Source: CAD feature listing. Evaluate the final solid. Frame: model axes, mm. A direction names the side the tool comes from. Give positions to 0.01 mm unless a question says otherwise; leave off trailing zeros. Loops run counter-clockwise (first coordinate to the right, second up) from the corner with the lowest first, then second, coordinate; pieces in that order, holes last. Notation, with made-up numbers: M -12.5,18 L 9.5,18 A14 cw 9.5,38 Z; hole C 86,29.25 d11. An arc over 180 degrees is marked long. Write item = value, one per line.
from build123d import *

# Parameters (mm, degrees)
BOSS_EXTRUDE1_DEPTH     = 13
SKETCH6_W               = 6
SKETCH6_H               = 5
BOSS_EXTRUDE4_DEPTH     = 5.6
SKETCH16_W              = 6
SKETCH16_H              = 8
BOSS_EXTRUDE5_DEPTH     = 0.1
CUT_EXTRUDE6_DEPTH      = 4
CUT_EXTRUDE6_DEPTH_BACK = 3.6
SKETCH15_R              = 1.2
CUT_EXTRUDE7_DEPTH      = 8.7202
CUT_EXTRUDE8_START      = -0.2202
SKETCH19_W              = 6
SKETCH19_H              = 8
SKETCH19_R              = 1.2
CUT_EXTRUDE8_DEPTH      = 0.2202
SKETCH12_R              = 1.2
CUT_EXTRUDE5_DEPTH      = 6
CHAMFER1_SIZE           = 0.2
SKETCH21_R              = 1.2
BOSS_EXTRUDE6_DEPTH     = 2.5
SKETCH24_W              = 6
SKETCH24_H              = 5.5
CUT_EXTRUDE10_DEPTH     = 8.5
SKETCH25_W              = 6
SKETCH25_H              = 7
BOSS_EXTRUDE8_DEPTH     = 12.9
SKETCH26_W              = 6
SKETCH26_H              = 7.39
BOSS_EXTRUDE9_DEPTH     = 3
SKETCH30_R              = 1.2
CUT_EXTRUDE13_DEPTH     = 8
SKETCH31_W              = 7
SKETCH31_H              = 9
BOSS_EXTRUDE11_DEPTH    = 1
SKETCH32_W              = 7
SKETCH32_H              = 9
BOSS_EXTRUDE12_DEPTH    = 1
BOSS_EXTRUDE13_DEPTH    = 1
BOSS_EXTRUDE14_DEPTH    = 1
SKETCH35_W              = 10
SKETCH35_H              = 4.2
CUT_EXTRUDE14_DEPTH     = 10
BOSS_EXTRUDE15_DEPTH    = 6
SKETCH38_R              = 1.2
CUT_EXTRUDE15_DEPTH     = 4
SKETCH39_R              = 1.2
CUT_EXTRUDE16_DEPTH     = 10
SKETCH40_W              = 14
SKETCH40_H              = 1.5
CUT_EXTRUDE17_DEPTH     = 10
SKETCH41_W              = 6.5
SKETCH41_H              = 3.19
CUT_EXTRUDE18_DEPTH     = 1.5


with BuildPart() as part:
    # Sketch1 → Boss-Extrude1 (new body)
    with BuildSketch(Plane.XY):
        Polygon((3, 3.05), (3, -2.253801214), (2.388188946, -2.95), (-2.388188946, -2.95), (-3, -2.253801214), (-3, 3.05), align=None)
    extrude(amount=BOSS_EXTRUDE1_DEPTH)

    # Sketch6 → Boss-Extrude4 (add)
    with BuildSketch(Plane(origin=(0, 3.05, 0), x_dir=(1, 0, 0), z_dir=(0, 1, 0))):
        with Locations((0, -2.5)):
            Rectangle(SKETCH6_W, SKETCH6_H)
    extrude(amount=BOSS_EXTRUDE4_DEPTH)

    # Sketch16 → Boss-Extrude5 (add)
    with BuildSketch(Plane(origin=(0, 3.05, 0), x_dir=(1, 0, 0), z_dir=(0, 1, 0))):
        with Locations((0, -9)):
            Rectangle(SKETCH16_W, SKETCH16_H)
    extrude(amount=BOSS_EXTRUDE5_DEPTH)

    # Sketch18 → Cut-Extrude6 (cut, two sides: drawn at the far end of the back side and taken through both)
    with BuildSketch(Plane(origin=(0, 0, 0), x_dir=(0, 0, -1), z_dir=(1, 0, 0)).offset(-CUT_EXTRUDE6_DEPTH_BACK)):
        with BuildLine():
            Line((-8.8572, -0.0702), (-12.8572, -0.0702))
            Line((-12.8572, -0.0702), (-13, -0.0702))
            Line((-13, -0.0702), (-13, -0.7))
            Line((-13, -0.7), (-12.8572, -0.7))
            Line((-12.8572, -0.7), (-12.7144, -0.7))
            add(Edge.make_bspline(
                [(-12.7144, -0.7), (-12.5198, -0.7), (-12.43, -0.9509)],
                knots=[0.103448276, 0.103448276, 0.103448276, 0.137931034, 0.137931034, 0.137931034], degree=2))
            add(Edge.make_bspline(
                [(-12.43, -0.9509), (-12.3594, -1.2388), (-12.13, -1.45), (-11.8572, -1.45)],
                knots=[0.137931034, 0.137931034, 0.137931034, 0.137931034, 0.172413793, 0.172413793, 0.172413793, 0.172413793], degree=3))
            add(Edge.make_bspline(
                [(-11.8572, -1.45), (-11.5844, -1.45), (-11.355, -1.2388), (-11.2844, -0.9509)],
                knots=[0.172413793, 0.172413793, 0.172413793, 0.172413793, 0.206896552, 0.206896552, 0.206896552, 0.206896552], degree=3))
            add(Edge.make_bspline(
                [(-11.2844, -0.9509), (-11.1946, -0.7), (-11, -0.7)],
                knots=[0.206896552, 0.206896552, 0.206896552, 0.24137931, 0.24137931, 0.24137931], degree=2))
            Line((-11, -0.7), (-10.8572, -0.7))
            Line((-10.8572, -0.7), (-10.7144, -0.7))
            add(Edge.make_bspline(
                [(-10.7144, -0.7), (-10.5198, -0.7), (-10.43, -0.9509)],
                knots=[0.310344828, 0.310344828, 0.310344828, 0.344827586, 0.344827586, 0.344827586], degree=2))
            add(Edge.make_bspline(
                [(-10.43, -0.9509), (-10.3594, -1.2388), (-10.13, -1.45), (-9.8572, -1.45)],
                knots=[0.344827586, 0.344827586, 0.344827586, 0.344827586, 0.379310345, 0.379310345, 0.379310345, 0.379310345], degree=3))
            add(Edge.make_bspline(
                [(-9.8572, -1.45), (-9.5844, -1.45), (-9.355, -1.2388), (-9.2844, -0.9509)],
                knots=[0.379310345, 0.379310345, 0.379310345, 0.379310345, 0.413793103, 0.413793103, 0.413793103, 0.413793103], degree=3))
            add(Edge.make_bspline(
                [(-9.2844, -0.9509), (-9.1946, -0.7), (-9, -0.7)],
                knots=[0.413793103, 0.413793103, 0.413793103, 0.448275862, 0.448275862, 0.448275862], degree=2))
            Line((-9, -0.7), (-8.8572, -0.7))
            Line((-8.8572, -0.7), (-8.7144, -0.7))
            add(Edge.make_bspline(
                [(-8.7144, -0.7), (-8.5198, -0.7), (-8.43, -0.9509)],
                knots=[0.517241379, 0.517241379, 0.517241379, 0.551724138, 0.551724138, 0.551724138], degree=2))
            add(Edge.make_bspline(
                [(-8.43, -0.9509), (-8.3594, -1.2388), (-8.13, -1.45), (-7.8572, -1.45)],
                knots=[0.551724138, 0.551724138, 0.551724138, 0.551724138, 0.586206897, 0.586206897, 0.586206897, 0.586206897], degree=3))
            add(Edge.make_bspline(
                [(-7.8572, -1.45), (-7.5844, -1.45), (-7.355, -1.2388), (-7.2844, -0.9509)],
                knots=[0.586206897, 0.586206897, 0.586206897, 0.586206897, 0.620689655, 0.620689655, 0.620689655, 0.620689655], degree=3))
            add(Edge.make_bspline(
                [(-7.2844, -0.9509), (-7.1946, -0.7), (-7, -0.7)],
                knots=[0.620689655, 0.620689655, 0.620689655, 0.655172414, 0.655172414, 0.655172414], degree=2))
            Line((-7, -0.7), (-6.8572, -0.7))
            Line((-6.8572, -0.7), (-6.7144, -0.7))
            add(Edge.make_bspline(
                [(-6.7144, -0.7), (-6.5198, -0.7), (-6.43, -0.9509)],
                knots=[0.724137931, 0.724137931, 0.724137931, 0.75862069, 0.75862069, 0.75862069], degree=2))
            add(Edge.make_bspline(
                [(-6.43, -0.9509), (-6.3594, -1.2388), (-6.13, -1.45), (-5.8572, -1.45)],
                knots=[0.75862069, 0.75862069, 0.75862069, 0.75862069, 0.793103448, 0.793103448, 0.793103448, 0.793103448], degree=3))
            add(Edge.make_bspline(
                [(-5.8572, -1.45), (-5.5844, -1.45), (-5.355, -1.2388), (-5.2844, -0.9509)],
                knots=[0.793103448, 0.793103448, 0.793103448, 0.793103448, 0.827586207, 0.827586207, 0.827586207, 0.827586207], degree=3))
            add(Edge.make_bspline(
                [(-5.2844, -0.9509), (-5.1946, -0.7), (-5, -0.7)],
                knots=[0.827586207, 0.827586207, 0.827586207, 0.862068966, 0.862068966, 0.862068966], degree=2))
            Line((-5, -0.7), (-5, -0.0702))
            Line((-5, -0.0702), (-8.8572, -0.0702))
        make_face()
    extrude(amount=CUT_EXTRUDE6_DEPTH + CUT_EXTRUDE6_DEPTH_BACK, mode=Mode.SUBTRACT)

    # Sketch15 → Cut-Extrude7 (cut)
    with BuildSketch(Plane(origin=(0, 8.65, 0), x_dir=(1, 0, 0), z_dir=(0, 1, 0))):
        with Locations(Location((0, -10.8572, 0), (0, 0, 180))):
            Circle(SKETCH15_R)
        with Locations(Location((0, -6.8572, 0), (0, 0, 180))):
            Circle(SKETCH15_R)
    extrude(amount=-CUT_EXTRUDE7_DEPTH, mode=Mode.SUBTRACT)

    # Sketch19 → Cut-Extrude8 (cut)
    with BuildSketch(Plane.XZ.offset(0.0702).offset(CUT_EXTRUDE8_START)):
        with Locations((0, 9)):
            Rectangle(SKETCH19_W, SKETCH19_H)
        with Locations(Location((0, 10.8572, 0), (0, 0, 180))):
            Circle(SKETCH19_R, mode=Mode.SUBTRACT)
        with Locations(Location((0, 6.8572, 0), (0, 0, 180))):
            Circle(SKETCH19_R, mode=Mode.SUBTRACT)
    extrude(amount=CUT_EXTRUDE8_DEPTH, mode=Mode.SUBTRACT)

    # Sketch12 → Cut-Extrude5 (cut)
    with BuildSketch(Plane.XY.offset(5)):
        with Locations((0, 5.85)):
            Circle(SKETCH12_R)
    extrude(amount=-CUT_EXTRUDE5_DEPTH, mode=Mode.SUBTRACT)

    # Chamfer1
    chamfer1_edges = [part.edges().sort_by_distance(p)[0] for p in [
        (-2.694094473, -2.601900607, 13),
        (0, -2.95, 13),
        (2.694094473, -2.601900607, 13),
        (3, 1.65, 13),
        (3, -1.476900607, 13),
        (-3, -1.476900607, 13),
        (-3, 1.65, 13),
    ]]
    chamfer(chamfer1_edges, length=CHAMFER1_SIZE)

    # Sketch21 → Boss-Extrude6 (add)
    with BuildSketch(Plane(origin=(0, 0, 0), x_dir=(-1, 0, 0), z_dir=(0, 0, -1))):
        Polygon((-2.388188946, -2.95), (2.388188946, -2.95), (3, -2.253801214), (3, 8.65), (-3, 8.65), (-3, -2.253801214), align=None)
        with Locations(Location((0, 5.85, 0), (0, 0, 180))):
            Circle(SKETCH21_R, mode=Mode.SUBTRACT)
    extrude(amount=BOSS_EXTRUDE6_DEPTH)

    # Sketch24 → Cut-Extrude10 (cut)
    with BuildSketch(Plane.XY.offset(5)):
        with Locations((0, 5.9)):
            Rectangle(SKETCH24_W, SKETCH24_H)
    extrude(amount=-CUT_EXTRUDE10_DEPTH, mode=Mode.SUBTRACT)

    # Sketch25 → Boss-Extrude8 (add)
    with BuildSketch(Plane(origin=(0, 3.15, 0), x_dir=(1, 0, 0), z_dir=(0, 1, 0))):
        with Locations((0, -1)):
            Rectangle(SKETCH25_W, SKETCH25_H)
    extrude(amount=BOSS_EXTRUDE8_DEPTH)

    # Sketch26 → Boss-Extrude9 (add)
    with BuildSketch(Plane(origin=(0, 0, -2.5), x_dir=(-1, 0, 0), z_dir=(0, 0, -1))):
        with Locations((0, 12.355)):
            Rectangle(SKETCH26_W, SKETCH26_H)
    extrude(amount=BOSS_EXTRUDE9_DEPTH)

    # Sketch30 → Cut-Extrude13 (cut)
    with BuildSketch(Plane(origin=(0, 0, -2.5), x_dir=(-1, 0, 0), z_dir=(0, 0, -1))):
        with Locations((0, 5.9)):
            Circle(SKETCH30_R)
    extrude(amount=-CUT_EXTRUDE13_DEPTH, mode=Mode.SUBTRACT)

    # Sketch31 → Boss-Extrude11 (add)
    with BuildSketch(Plane(origin=(3, 0, 0), x_dir=(0, 0, -1), z_dir=(1, 0, 0))):
        with Locations((-1, 7.65)):
            Rectangle(SKETCH31_W, SKETCH31_H)
    extrude(amount=BOSS_EXTRUDE11_DEPTH)

    # Sketch32 → Boss-Extrude12 (add)
    with BuildSketch(Plane.ZY.offset(3)):
        with Locations((1, 7.65)):
            Rectangle(SKETCH32_W, SKETCH32_H)
    extrude(amount=BOSS_EXTRUDE12_DEPTH)

    # Sketch33 → Boss-Extrude13 (add)
    with BuildSketch(Plane(origin=(3, 0, 0), x_dir=(0, 0, -1), z_dir=(1, 0, 0))):
        Polygon((2.5, 12.15), (2.5, 8.66), (5.5, 8.66), (5.5, 16.05), (-4.5, 16.05), (-4.5, 12.15), align=None)
    extrude(amount=BOSS_EXTRUDE13_DEPTH)

    # Sketch34 → Boss-Extrude14 (add)
    with BuildSketch(Plane.ZY.offset(3)):
        Polygon((-2.5, 12.15), (4.5, 12.15), (4.5, 16.05), (-5.5, 16.05), (-5.5, 8.66), (-2.5, 8.66), align=None)
    extrude(amount=BOSS_EXTRUDE14_DEPTH)

    # Sketch35 → Cut-Extrude14 (cut)
    with BuildSketch(Plane.ZY.offset(4)):
        with Locations((-0.5, 13.95)):
            Rectangle(SKETCH35_W, SKETCH35_H)
    extrude(amount=-CUT_EXTRUDE14_DEPTH, mode=Mode.SUBTRACT)

    # Sketch36 → Boss-Extrude15 (add)
    with BuildSketch(Plane.ZY.offset(4)):
        Polygon((4.5, 3.15), (4.5, 11.85), (-5.5, 11.85), (-5.5, 8.66), (-2.5, 8.66), (-2.5, 3.15), align=None)
    extrude(amount=BOSS_EXTRUDE15_DEPTH)

    # Sketch38 → Cut-Extrude15 (cut)
    with BuildSketch(Plane(origin=(0, 11.85, 0), x_dir=(1, 0, 0), z_dir=(0, 1, 0))):
        with Locations(Location((0.5, -1, 0), (0, 0, 270))):
            Circle(SKETCH38_R)
    extrude(amount=-CUT_EXTRUDE15_DEPTH, mode=Mode.SUBTRACT)

    # Sketch39 → Cut-Extrude16 (cut)
    with BuildSketch(Plane(origin=(0, 11.85, 0), x_dir=(1, 0, 0), z_dir=(0, 1, 0))):
        with Locations(Location((-6.5, -1, 0), (0, 0, 270))):
            Circle(SKETCH39_R)
    extrude(amount=-CUT_EXTRUDE16_DEPTH, mode=Mode.SUBTRACT)

    # Sketch40 → Cut-Extrude17 (cut)
    with BuildSketch(Plane(origin=(0, 11.85, 0), x_dir=(1, 0, 0), z_dir=(0, 1, 0))):
        with Locations((-3, 4.75)):
            Rectangle(SKETCH40_W, SKETCH40_H)
    extrude(amount=-CUT_EXTRUDE17_DEPTH, mode=Mode.SUBTRACT)

    # Sketch41 → Cut-Extrude18 (cut)
    with BuildSketch(Plane(origin=(0, 0, -4), x_dir=(-1, 0, 0), z_dir=(0, 0, -1))):
        with Locations((6.75, 10.255)):
            Rectangle(SKETCH41_W, SKETCH41_H)
    extrude(amount=-CUT_EXTRUDE18_DEPTH, mode=Mode.SUBTRACT)


solid = part.part
1. First-contact query: pin 1 Ø2 at (x, y) = (-1, 8.5) entering from +Z; pin 2 Ø3.5 at (x, z) = (-8, 2.5) entering from -Y; pin 3 Ø7 at (x, y) = (-5, 5) entering from -Z; pin 4 Ø2 at (x, y) = (0, 5.9) entering from -Z. Flat tips, straight axial feed; report the tip coordinate or a pass-through.
Derived:
pin_1 = 4.5
pin_2 = 3.15
pin_3 = -2.5
pin_4 = through
2. Cut plane C-C, the plane x = -6.5. Return the cut outline in (y, z).
Derived:
outline = M 3.15,-2.5 L 11.85,-2.5 L 11.85,-0.2 L 3.15,-0.2 Z; M 3.15,2.2 L 11.85,2.2 L 11.85,4.5 L 3.15,4.5 Z
3. Pull-direction query (Z, two-part tool) for faces 6 (the flat face through (1, 7.85, 1)), 7 (the flat face through (0, -2, 13)), 8 (the flat face through (4, 8, 1)); classes: +Z half, -Z half, draft (parallel to the pull), parting line (faces both ways), or undercut.
Derived:
face_6 = undercut
face_7 = +Z half
face_8 = draft
4. Cut plane D-D, the plane z = -1.25. Return the cut outline in (x, y), then the cut area to 3 significant figures.
Derived:
outline = M -10,3.15 L -3,3.15 L -3,-2.25 L -2.39,-2.95 L 2.39,-2.95 L 3,-2.25 L 3,3.15 L 4,3.15 L 4,11.85 L -10,11.85 Z; hole C 0,5.9 d2.4
area = 153 mm²
5. Material intervals for probe 1 along X at (y, z) = (10.5, 1); probe 2 along Z at (x, y) = (0, 2.15); probe 3 along Y at (x, z) = (0, 1.5), sorted ascending. Write a range as from..to.
Derived:
probe_1 = -10..-7.7, -5.3..-0.7, 1.7..4
probe_2 = -2.5..5.66, 8.06..9.66, 12.06..13
probe_3 = -2.95..4.7, 7.1..7.85
6. Cut plane A-A, the plane y = 5.9. Return the cut outline in (x, z), then the cut area to 3 significant figures.
Derived:
outline = M -10,-2.5 L -1.2,-2.5 L -1.2,4.5 L -10,4.5 Z; M 1.2,-2.5 L 4,-2.5 L 4,4.5 L 1.2,4.5 Z; hole C -6.5,1 d2.4
area = 76.7 mm²
7. Reachability of faces 1 (the flat face through (0, 8.66, -3)), 2 (the flat face through (0, 0, 5)), 3 (the flat face through (-3, 7, 4.5)), 4 (the flat face through (-3, 0.4, 5.3)), 5 (the cylindrical face through (0.26, 1.671, 9.686)) from +Z, -Z, +X, -X, +Y, -Y: full face, straight path, thin tool, end or side. Return the list, or none.
Derived:
face_1 = -Z, +X, -X, -Y
face_2 = +Z, +X, -X
face_3 = +Z, +X, -X, +Y
face_4 = +Z, -Z, -X, -Y
face_5 = +Y
8. Cut plane B-B, the plane z = 1. Return the cut outline in (x, y), then the cut area to 3 significant figures.
Derived:
outline = M -10,3.15 L -7.7,3.15 L -7.7,11.85 L -10,11.85 Z; M -5.3,3.15 L -3,3.15 L -3,-2.25 L -2.39,-2.95 L 2.39,-2.95 L 3,-2.25 L 3,3.15 L 4,3.15 L 4,11.85 L 1.7,11.85 L 1.7,7.85 L -0.7,7.85 L -0.7,11.85 L -5.3,11.85 Z; hole C 0,5.9 d2.4
area = 123 mm²
